Source: CAD feature listing. Evaluate the final solid. Frame: model axes, mm. Round coordinates to 2 decimals unless told otherwise and drop trailing zeros. Order: outer loops, then holes, each group sorted by start corner. A loop starts at its lowest first (then second) coordinate and runs counter-clockwise, first axis right, second up. Notation, with made-up numbers: (43.25, 3) -> (86.25, 3) arc R29 ccw to (86.25, 29) -> close; hole circle Ø5 at (-34, 17). An arc over 180 degrees is marked (long way). Answer as CSV lines item,"result". Start each with the question number.
(1) Line query: line 1 along X through (y, z) = (0.95, 13.7); line 2 along X through (y, z) = (1.35, 13). Output: solid intervals per line, ascending. Write a range as from..to.
(2) Contact query for a flat-ended pin moving along its axis: P1, Ø1.4, axis at x = 33.5, z = 14.5, coming from the +Y side. Output: stop coordinate, or through.
(3) Section query A-A (z = 13.7). Output: boundary loops of the cut face in (x, y), plus the area to 3 significant figures.
(4) Section query B-B (y = 0.5). Output: boundary loops of the cut face in (x, z).
```python
from build123d import *

# Parameters (mm, degrees)
SKETCH_1_W          = 74
SKETCH_1_H          = 35.6
EXTRUDE_1_DEPTH     = 2
CHAMFER_1_SIZE      = 1
SKETCH_2_R          = 1.2
CUT_EXTRUDE_1_DEPTH = 42.107663519
SKETCH_3_R          = 2.4
CUT_EXTRUDE_2_DEPTH = 0.6
SKETCH_5_W          = 8
SKETCH_5_H          = 5
CUT_EXTRUDE_3_DEPTH = 42.107663519
FILLET_1_R          = 4.4


with BuildPart() as part:
    # 草图1 → 凸台-拉伸1 (new body)
    with BuildSketch(Plane(origin=(0, 0, 0), x_dir=(1, 0, 0), z_dir=(0, 1, 0))):
        Rectangle(SKETCH_1_W, SKETCH_1_H)
    extrude(amount=EXTRUDE_1_DEPTH)

    # 倒角1
    chamfer_1_edges = [part.edges().sort_by_distance(p)[0] for p in [
        (37, 1, 17.8),
        (-37, 1, 17.8),
    ]]
    chamfer(chamfer_1_edges, length=CHAMFER_1_SIZE)

    # 草图2 → 切除-拉伸1 (cut, through all)
    with BuildSketch(Plane(origin=(0, 2, 0), x_dir=(1, 0, 0), z_dir=(0, 1, 0))):
        with Locations(Location((32.904560765, -13.813886845, 0), (0, 0, 270))):
            Circle(SKETCH_2_R)
        with Locations(Location((-32.9, -13.7, 0), (0, 0, 270))):
            Circle(SKETCH_2_R)
        with Locations(Location((-32.9, 13.799098008, 0), (0, 0, 270))):
            Circle(SKETCH_2_R)
        with Locations(Location((32.9, 13.799098008, 0), (0, 0, 270))):
            Circle(SKETCH_2_R)
    extrude(amount=-CUT_EXTRUDE_1_DEPTH, mode=Mode.SUBTRACT)

    # 草图3 → 切除-拉伸2 (cut)
    with BuildSketch(Plane(origin=(0, 2, 0), x_dir=(1, 0, 0), z_dir=(0, 1, 0))):
        with Locations(Location((32.904560765, -13.813886845, 0), (0, 0, 270))):
            Circle(SKETCH_3_R)
        with Locations(Location((-32.9, -13.7, 0), (0, 0, 270))):
            Circle(SKETCH_3_R)
        with Locations(Location((32.9, 13.799098008, 0), (0, 0, 270))):
            Circle(SKETCH_3_R)
        with Locations(Location((-32.9, 13.799098008, 0), (0, 0, 270))):
            Circle(SKETCH_3_R)
    extrude(amount=-CUT_EXTRUDE_2_DEPTH, mode=Mode.SUBTRACT)

    # 草图5 → 切除-拉伸3 (cut, through all)
    with BuildSketch(Plane(origin=(0, 2, 0), x_dir=(1, 0, 0), z_dir=(0, 1, 0))):
        with Locations((-24.9, 15.3)):
            Rectangle(SKETCH_5_W, SKETCH_5_H)
    extrude(amount=-CUT_EXTRUDE_3_DEPTH, mode=Mode.SUBTRACT)

    # 圆角1
    fillet_1_edges = [part.edges().sort_by_distance(p)[0] for p in [
        (-20.9, 1, -17.8),
        (-28.9, 1, -17.8),
    ]]
    fillet(fillet_1_edges, radius=FILLET_1_R)


solid = part.part
```
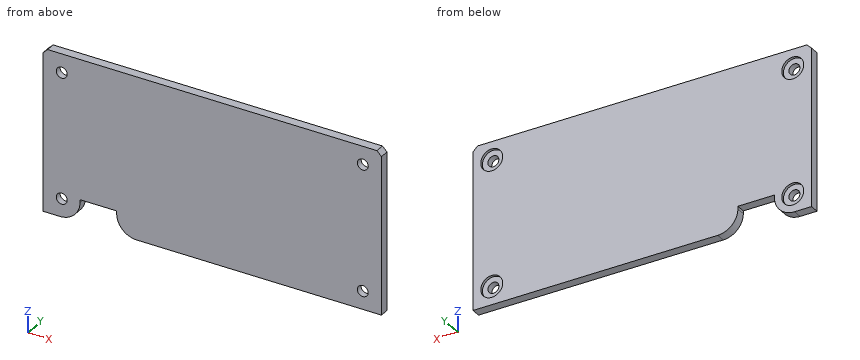
Answer block:
1,line 1,"-37..-34.1, -31.7..31.71, 34.1..37"
1,line 2,"-37..-33.87, -31.93..32.02, 33.79..37"
2,P1,"y = 1.4"
3,outline,"(-37, 0) -> (-34.1, 0) -> (-34.1, 1.4) -> (-35.3, 1.4) -> (-35.3, 2) -> (-37, 2) -> close; (-31.7, 0) -> (31.71, 0) -> (31.71, 1.4) -> (30.51, 1.4) -> (30.51, 2) -> (-30.5, 2) -> (-30.5, 1.4) -> (-31.7, 1.4) -> close; (34.1, 0) -> (37, 0) -> (37, 2) -> (35.3, 2) -> (35.3, 1.4) -> (34.1, 1.4) -> close"
3,area,"136 mm2"
4,outline,"(-37, -17.8) -> (-33.3, -17.8) arc R4.4 ccw to (-28.9, -13.4) -> (-28.9, -12.8) -> (-20.9, -12.8) -> (-20.9, -13.4) arc R4.4 ccw to (-16.5, -17.8) -> (37, -17.8) -> (37, 16.8) -> (36, 17.8) -> (-36, 17.8) -> (-37, 16.8) -> close; hole circle Ø2.4 at (-32.9, -13.8); hole circle Ø2.4 at (-32.9, 13.7); hole circle Ø2.4 at (32.9, -13.8); hole circle Ø2.4 at (32.9, 13.81)"
